Job drawing, mm, ordinate dimensions from the low corner. One solid piece. A direction names the side the tool comes from. Coordinates: 2 decimals unless noted, no trailing zeros. Loops run counter-clockwise (first coordinate to the right, second up) from the corner with the lowest first, then second, coordinate; pieces in that order, holes last. Notation, with made-up numbers: (-37, -12.5) -> (-1, -12.5) arc R19 cw to (-1, 12.5) -> close; hole circle Ø8 at (32.25, 35.25). An arc over 180 degrees is marked (long way). Answer as CSV lines item,"result". Start each with the question number.
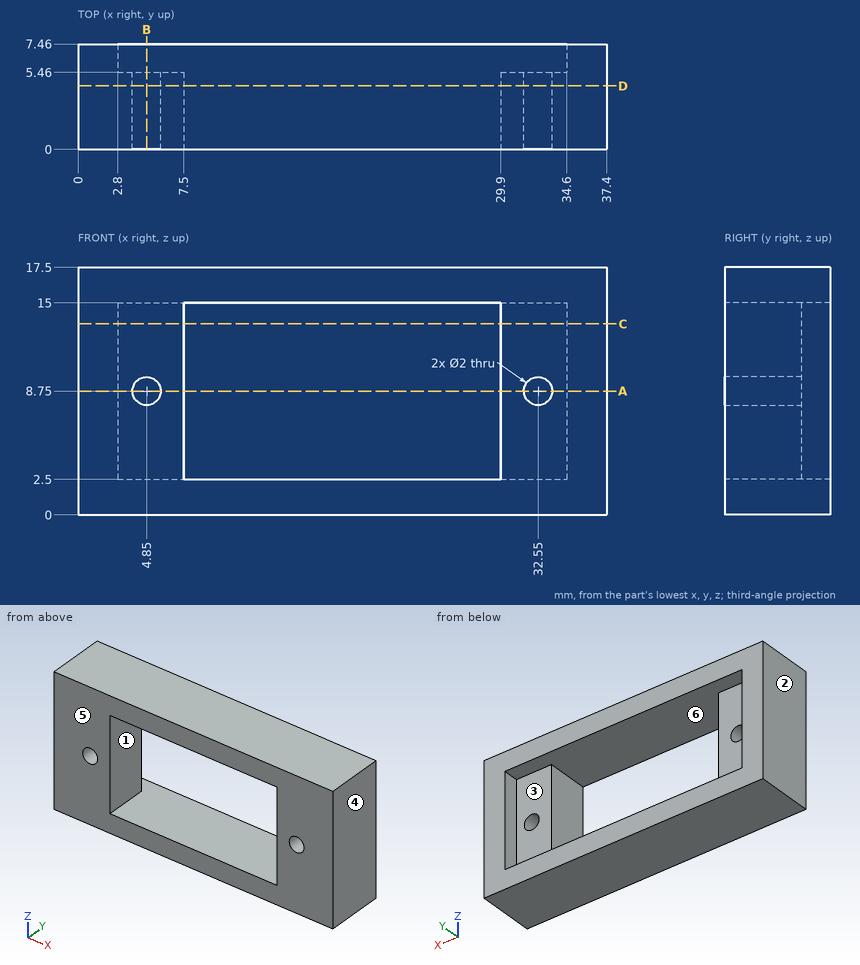
Q1. Probe probe 1 along X at (y, z) = (2.15, 8.75); probe 2 along X at (y, z) = (4.75, 11); probe 3 along X at (y, z) = (5.75, 11.5). List the from-to ranges inside material, lowest first. Write a range as from..to.
Q2. Saw through at B-B (x = 4.85). List the corners of the cut face in (y, z).
Q3. Pin check, flat tip, straight feed: pin 1 Ø3 at (x, z) = (32.55, 8.75) entering from +Y. Stop position of the tip, or through.
Q4. Saw through at C-C (z = 13.5). List the corners of the cut face in (x, y).
Q5. Which spindle directions (+Z, -Z, +X, -X, +Y, -Y) get a long thin tool onto all of the face, cutting with end or side? Do the marked faces 1, 2 and 3. Say none if no direction does.
Q6. Saw through at D-D (y = 4.5). List the corners of the cut face in (x, z), and give its area (3 significant figures).
Q7. Two-plate mould, pull along X, no slides. Class the marked faces 4, 5 and 6: pulls with the +X half, pulls with the -X half, needs draft (parallel to the pull), parting line crosses it, or undercut.
Q8. Saw through at A-A (z = 8.75). List the corners of the cut face in (x, y), and give its area (3 significant figures).
Ans:
1,probe 1,"x = 0..3.85, 5.85..7.5, 29.9..31.55, 33.55..37.4"
1,probe 2,"x = 0..7.5, 29.9..37.4"
1,probe 3,"x = 0..2.8, 34.6..37.4"
2,outline,"(0, 0) -> (7.46, 0) -> (7.46, 2.5) -> (5.46, 2.5) -> (5.46, 7.75) -> (0, 7.75) -> close; (0, 9.75) -> (5.46, 9.75) -> (5.46, 15) -> (7.46, 15) -> (7.46, 17.5) -> (0, 17.5) -> close"
3,pin 1,"stops at y = 5.46"
4,outline,"(0, 0) -> (7.5, 0) -> (7.5, 5.46) -> (2.8, 5.46) -> (2.8, 7.46) -> (0, 7.46) -> close; (29.9, 0) -> (37.4, 0) -> (37.4, 7.46) -> (34.6, 7.46) -> (34.6, 5.46) -> (29.9, 5.46) -> close"
5,face 1,"+Y, -Y"
5,face 2,"+Z, -Z, -X, +Y, -Y"
5,face 3,"+Y"
6,outline,"(0, 0) -> (37.4, 0) -> (37.4, 17.5) -> (0, 17.5) -> close; hole circle Ø2 at (4.85, 8.75); hole (7.5, 2.5) -> (29.9, 2.5) -> (29.9, 15) -> (7.5, 15) -> close; hole circle Ø2 at (32.55, 8.75)"
6,area,"368 mm²"
7,face 4,"pulls with the +X half"
7,face 5,"needs draft"
7,face 6,"undercut"
8,outline,"(0, 0) -> (3.85, 0) -> (3.85, 5.46) -> (2.8, 5.46) -> (2.8, 7.46) -> (0, 7.46) -> close; (5.85, 0) -> (7.5, 0) -> (7.5, 5.46) -> (5.85, 5.46) -> close; (29.9, 0) -> (31.55, 0) -> (31.55, 5.46) -> (29.9, 5.46) -> close; (33.55, 0) -> (37.4, 0) -> (37.4, 7.46) -> (34.6, 7.46) -> (34.6, 5.46) -> (33.55, 5.46) -> close"
8,area,"71.3 mm²"
